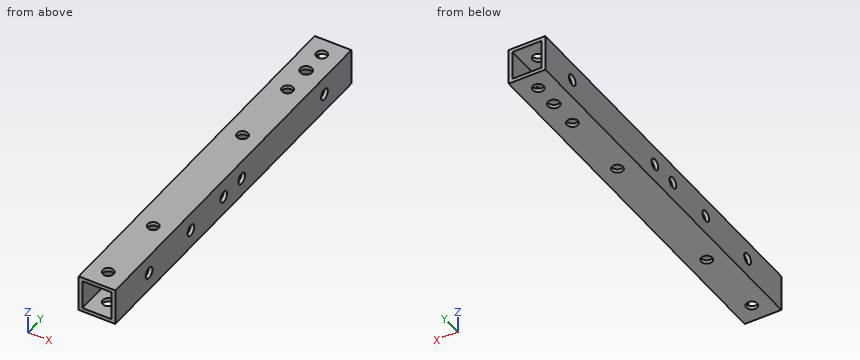
from build123d import *

# Parameters (mm, degrees)
SKETCH_1_W          = 10
SKETCH_1_H          = 10
SKETCH_1_W_2        = 8
SKETCH_1_H_2        = 8
EXTRUDE_1_DEPTH     = 104.9
SKETCH_2_R          = 1.5
SKETCH_2_R_2        = 1.6
CUT_EXTRUDE_1_DEPTH = 106.494123059
SKETCH_3_R          = 1.5
CUT_EXTRUDE_2_DEPTH = 106.494123059


with BuildPart() as part:
    # ｽｹｯﾁ1 → 押し出し-薄板1 (new body)
    with BuildSketch(Plane(origin=(0, 0, 0), x_dir=(1, 0, 0), z_dir=(0, 1, 0))):
        Rectangle(SKETCH_1_W, SKETCH_1_H)
        Rectangle(SKETCH_1_W_2, SKETCH_1_H_2, mode=Mode.SUBTRACT)
    extrude(amount=EXTRUDE_1_DEPTH)

    # ｽｹｯﾁ2 → ｶｯﾄ - 押し出し1 (cut, through all)
    with BuildSketch(Plane.XY.offset(5)):
        with Locations((0, 5)):
            Circle(SKETCH_2_R)
        with Locations((0, 64.7)):
            Circle(SKETCH_2_R)
        with Locations((0, 99.9)):
            Circle(SKETCH_2_R)
        with Locations((0, 84.7)):
            Circle(SKETCH_2_R)
        with Locations((0, 25)):
            Circle(SKETCH_2_R)
        with Locations((0, 92.95)):
            Circle(SKETCH_2_R_2)
    extrude(amount=-CUT_EXTRUDE_1_DEPTH, mode=Mode.SUBTRACT)

    # ｽｹｯﾁ3 → ｶｯﾄ - 押し出し2 (cut, through all)
    with BuildSketch(Plane(origin=(5, 0, 0), x_dir=(0, 0, -1), z_dir=(1, 0, 0))):
        with Locations((0, 33.6)):
            Circle(SKETCH_3_R)
        with Locations((0, 15)):
            Circle(SKETCH_3_R)
        with Locations((0, 48.2)):
            Circle(SKETCH_3_R)
        with Locations((0, 56.2)):
            Circle(SKETCH_3_R)
        with Locations((0, 92.95)):
            Circle(SKETCH_3_R)
    extrude(amount=-CUT_EXTRUDE_2_DEPTH, mode=Mode.SUBTRACT)


solid = part.part
Source: CAD feature listing. Evaluate the final solid. Frame: model axes, mm. Coordinates: 2 decimals unless noted, no trailing zeros. Loops run counter-clockwise (first coordinate to the right, second up) from the corner with the lowest first, then second, coordinate; pieces in that order, holes last. Notation, with made-up numbers: (-9, 88.5) - (1, 88.5) arc R17 ccw to (1, 97.5) - close; hole circle Ø5 at (18, 73). An arc over 180 degrees is marked (long way). One line per item, written item: value. Start each with the question number.
1. Contact query for a flat-ended pin moving along its axis: P1, Ø4, axis at x = 0, y = 25, coming from the +Z side. Output: stop coordinate, or through.
2. Section B-B (x = -3). Return the cut outline in (y, z).
3. Section C-C (y = 92.95). Return the cut outline in (x, z), and give its area (3 significant figures).
4. Section D-D (y = 38.5). Return the cut outline in (x, z).
5. Ray query, L1, parallel to Y at x = 4.75, z = 0; L2, parallel to X at y = 45.5, z = 0. Return the intervals inside material, ascending.
6. Section A-A (y = 5). Return the cut outline in (x, z).
Verdict:
1. P1: stops at z = 5
2. outline: (0, -5) - (104.9, -5) - (104.9, -4) - (0, -4) - close; (0, 4) - (104.9, 4) - (104.9, 5) - (0, 5) - close
3. outline: (-5, -5) - (-1.6, -5) - (-1.6, -4) - (-4, -4) - (-4, -1.5) - (-5, -1.5) - close; (-5, 1.5) - (-4, 1.5) - (-4, 4) - (-1.6, 4) - (-1.6, 5) - (-5, 5) - close; (1.6, -5) - (5, -5) - (5, -1.5) - (4, -1.5) - (4, -4) - (1.6, -4) - close; (1.6, 4) - (4, 4) - (4, 1.5) - (5, 1.5) - (5, 5) - (1.6, 5) - close
3. area: 23.6 mm2
4. outline: (-5, -5) - (5, -5) - (5, 5) - (-5, 5) - close; hole (-4, -4) - (4, -4) - (4, 4) - (-4, 4) - close
5. L1: y = 0 to 13.5, 16.5 to 32.1, 35.1 to 46.7, 49.7 to 54.7, 57.7 to 91.45, 94.45 to 104.9
5. L2: x = -5 to -4, 4 to 5
6. outline: (-5, -5) - (-1.5, -5) - (-1.5, -4) - (-4, -4) - (-4, 4) - (-1.5, 4) - (-1.5, 5) - (-5, 5) - close; (1.5, -5) - (5, -5) - (5, 5) - (1.5, 5) - (1.5, 4) - (4, 4) - (4, -4) - (1.5, -4) - close
